Geometry: see drawing. Coordinates: mm, zero at the bounding-box minimum. A direction names the side the tool comes from. Give positions to 0.01 mm unless a question says otherwise; leave off trailing zeros. Loops run counter-clockwise (first coordinate to the right, second up) from the corner with the lowest first, then second, coordinate; pieces in that order, holes last. Notation, with made-up numbers: (46, 2) -> (68, 2) arc R20 cw to (68, 36) -> close; hole circle Ø4 at (-32.75, -27). An arc over 180 degrees is marked (long way). Return JSON: item names as keys, results as strings. Group by question number.
(1) Access query for the marked faces 5 and 6. Directions: +Z, -Z, +X, -X, +Y, -Y. A direction counts if a zero-diameter tool reaches every point of the face in a straight line with its end or side. Return the directions, or none.
(2) Pin query (flat end, axial travel): pin 1 (3 mm diameter, centred on y = 4, z = 53, fed in from -X); pin 2 (3 mm diameter, centred on x = 26, y = 2, fed in from +Z); pin 3 (3 mm diameter, centred on y = 4, z = 54.5, fed in from +X). Return the tip coordinate at first contact, or that it passes through.
(3) Cut plane A-A on z = 8.5. Return loops of the section in (x, y).
(4) Ray query, line 1 (X direction, y = 5, z = 52.5); line 2 (X direction, y = 4.25, z = 8.5); line 3 (Z direction, x = 24.5, y = 6.25). Return the intervals inside material, ascending. Write a range as from..to.
(5) Cut plane B-B on z = 31. Return loops of the section in (x, y).
(6) Cut plane C-C on y = 1. Give the number of separate pieces and of enclosed holes in the cut face, then the cut area to 3 significant figures.
(7) Draft query along Z for the marked faces 1, 2, 3 and 4. Return one class per face: released by +Z, released by -Z, zero draft, split by the parting line, or undercut.
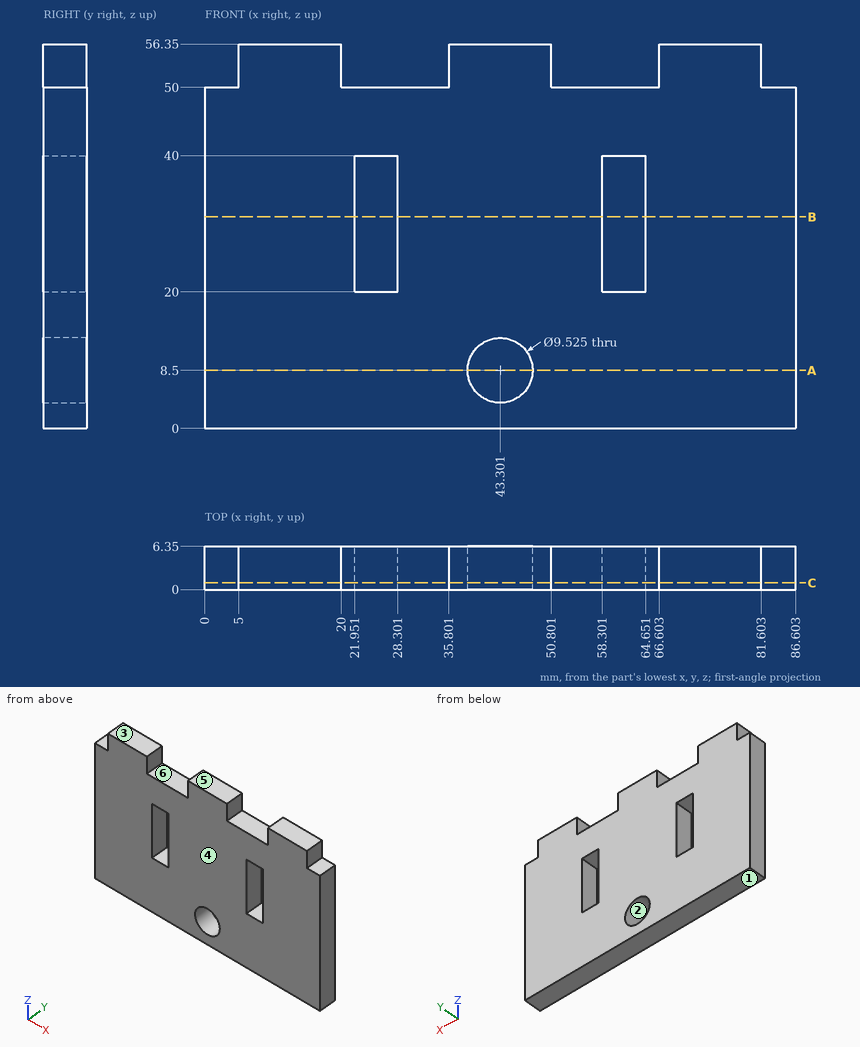
Answers:
{
 "1": {"face 5": "+Z, +X, -X, +Y, -Y", "face 6": "+Z, +Y, -Y"},
 "2": {"pin 1": "x = 5", "pin 2": "z = 50", "pin 3": "x = 81.6"},
 "3": {"outline": "(0, 0) -> (38.54, 0) -> (38.54, 6.35) -> (0, 6.35) -> close; (48.06, 0) -> (86.6, 0) -> (86.6, 6.35) -> (48.06, 6.35) -> close"},
 "4": {"line 1": "5..20, 35.8..50.8, 66.6..81.6", "line 2": "0..38.54, 48.06..86.6", "line 3": "0..20, 40..50"},
 "5": {"outline": "(0, 0) -> (21.95, 0) -> (21.95, 6.35) -> (0, 6.35) -> close; (28.3, 0) -> (58.3, 0) -> (58.3, 6.35) -> (28.3, 6.35) -> close; (64.65, 0) -> (86.6, 0) -> (86.6, 6.35) -> (64.65, 6.35) -> close"},
 "6": {"separate pieces": "1", "enclosed holes": "3", "area": "4,290 mm²"},
 "7": {"face 1": "released by -Z", "face 2": "undercut", "face 3": "released by +Z", "face 4": "zero draft"}
}
